```python
from build123d import *

# Parameters (mm, degrees)
SKETCH1_R           = 12.7
SKETCH1_R_2         = 9.75
BOSS_EXTRUDE1_DEPTH = 123
SKETCH7_R           = 1.5
SKETCH7_R_2         = 2
CUT_EXTRUDE1_DEPTH  = 108
BOSS_EXTRUDE2_START = 4.17
SKETCH8_R           = 12.7
SKETCH8_R_2         = 9.75
BOSS_EXTRUDE2_DEPTH = 4.17


with BuildPart() as part:
    # Sketch1 → Boss-Extrude1 (new body)
    with BuildSketch(Plane.XY):
        Circle(SKETCH1_R)
        Circle(SKETCH1_R_2, mode=Mode.SUBTRACT)
    extrude(amount=BOSS_EXTRUDE1_DEPTH)

    # Sketch7 → Cut-Extrude1 (cut)
    with BuildSketch(Plane(origin=(0, 0, 0), x_dir=(1, 0, 0), z_dir=(0, 1, 0))):
        with Locations(Location((0, -10.17, 0), (0, 0, 270))):
            Circle(SKETCH7_R)
        with Locations(Location((0, -29, 0), (0, 0, 270))):
            Circle(SKETCH7_R)
        with Locations(Location((0, -113, 0), (0, 0, 270))):
            Circle(SKETCH7_R_2)
    extrude(amount=-CUT_EXTRUDE1_DEPTH, mode=Mode.SUBTRACT)

    # Sketch8 → Boss-Extrude2 (add)
    with BuildSketch(Plane(origin=(0, 0, 0), x_dir=(-1, 0, 0), z_dir=(0, 0, -1)).offset(BOSS_EXTRUDE2_START)):
        Circle(SKETCH8_R)
        Circle(SKETCH8_R_2, mode=Mode.SUBTRACT)
    extrude(amount=-BOSS_EXTRUDE2_DEPTH)


solid = part.part
```
Geometry: final body of the model. Coordinates: model frame, mm. Coordinates: 2 decimals unless noted, no trailing zeros. Order: outer loops, then holes, each group sorted by start corner. A loop starts at its lowest first (then second) coordinate and runs counter-clockwise, first axis right, second up. Notation, with made-up numbers: M 14,57.5 L 72,57.5 A21 ccw 72,66.5 Z; hole C 48,15.5 d6. An arc over 180 degrees is marked long. Answer in a Markdown table with one row per item. Add a question column.
Q1. Section query D-D on x = -7.75. Return the cut outline in (y, z).
Q2. Section query A-A on x = 0. Return the cut outline in (y, z).
Q3. Section query C-C on z = 101.5. Return the cut outline in (x, y), and give its area (3 significant figures).
Q4. Line query: L1, parallel to Z at x = 0, y = -11.25; L2, parallel to Y at x = -0.5, z = 54; L3, parallel to X at y = 0.25, z = 19. Output: solid intervals per line, ascending.
Q5. Section query B-B on y = 0. Return the cut outline in (x, z).
Q6. Mould query, pull axis Z, two halves, no side actions, for faces 1 (the flat face through (-3.7, -9.3, -4.17)), 2 (the flat face through (3.7, -9.3, 123)), 3 (the cylindrical face through (0, -11, 111)). Classes: released by +Z, released by -Z, zero draft, split by the parting line, or undercut.
Q7. Contact query for flat-ended pins moving along their axis: P1, Ø1.5, axis at y = -5, z = 62, coming from the -X side; P2, Ø2, axis at x = -2.5, z = 63.5, coming from the -Y side; P3, Ø1, axis at x = 1.5, z = 94, coming from the -Y side. Output: stop coordinate, or through.
Completed:
| question | item | result |
|---|---|---|
| 1 | outline | M -10.06,-4.17 L -5.92,-4.17 L -5.92,123 L -10.06,123 Z; M 5.92,-4.17 L 10.06,-4.17 L 10.06,123 L 5.92,123 Z |
| 2 | outline | M -12.7,-4.17 L -9.75,-4.17 L -9.75,8.67 L -12.7,8.67 Z; M -12.7,11.67 L -9.75,11.67 L -9.75,27.5 L -12.7,27.5 Z; M -12.7,30.5 L -9.75,30.5 L -9.75,111 L -12.7,111 Z; M -12.7,115 L -9.75,115 L -9.75,123 L -12.7,123 Z; M 9.75,-4.17 L 12.7,-4.17 L 12.7,123 L 9.75,123 Z |
| 3 | outline | C 0,0 d25.4; hole C 0,0 d19.5 |
| 3 | area | 208 mm2 |
| 4 | L1 | z = -4.17 to 8.67, 11.67 to 27.5, 30.5 to 111, 115 to 123 |
| 4 | L2 | y = -12.69 to -9.74, 9.74 to 12.69 |
| 4 | L3 | x = -12.7 to -9.75, 9.75 to 12.7 |
| 5 | outline | M -12.7,-4.17 L -9.75,-4.17 L -9.75,123 L -12.7,123 Z; M 9.75,-4.17 L 12.7,-4.17 L 12.7,123 L 9.75,123 Z |
| 6 | face 1 | released by -Z |
| 6 | face 2 | released by +Z |
| 6 | face 3 | undercut |
| 7 | P1 | stops at x = -11.97 |
| 7 | P2 | stops at y = -12.61 |
| 7 | P3 | stops at y = -12.66 |
